from build123d import *

# Parameters (mm, degrees)
F0_W     = 48.26
F0_H     = 73.66
F1_DEPTH = 48.26
F3_DEPTH = 30.48
F5_DEPTH = 30.48
F7_DEPTH = 25.4
F8_W     = 3.175
F8_H     = 3.175
F9_DEPTH = 19.05


with BuildPart() as f1:
    # F0 (on Top) → F1 (new body)
    with BuildSketch(Plane.XY):
        with Locations((24.13, 36.83)):
            Rectangle(F0_W, F0_H)
    extrude(amount=F1_DEPTH)

    # F2 (on face) → F3 (join)
    with BuildSketch(Plane(origin=(0, 73.66, 0), x_dir=(-1, 0, 0), z_dir=(0, 1, 0))):
        Polygon((-12.1206499105, 44.9308045208), (-24.13, 44.9308045208), (-24.13, 24.13), (-24.13, 9.0534836054), (-48.0858952621, 24.0212186931), (-36.1393500895, 3.3291954792), (-12.1206499105, 3.3291954792), (-0.1112998211, 24.13), align=None)
        Polygon((-24.13, 24.13), (-24.13, 44.9308045208), (-36.1393500895, 44.9308045208), (-48.1487001789, 24.13), align=None)
        Polygon((-24.13, 9.0534836054), (-24.13, 24.13), (-48.1487001789, 24.13), (-48.0858952621, 24.0212186931), align=None)
        Polygon((-48.0858952621, 24.0212186931), (-48.1487001789, 24.13), (-48.26, 24.13), align=None)
    extrude(amount=F3_DEPTH)

    # F4 (on face) → F5 (join)
    with BuildSketch(Plane(origin=(0, 104.14, 0), x_dir=(-1, 0, 0), z_dir=(0, 1, 0))):
        Polygon((-15.8659655868, 38.4132767837), (-24.13, 38.4209016232), (-24.13, 24.0781502233), (-7.6297935663, 24.1173632016), align=None)
        Polygon((-24.13, 24.0781502233), (-24.13, 38.4209016232), (-32.3676633374, 38.4285021314), (-40.6316977506, 24.1452253477), (-40.5705446588, 24.0390790321), align=None)
        Polygon((-7.6297935663, 24.1173632016), (-24.13, 24.0781502233), (-24.13, 9.8390983768), (-15.8923366626, 9.8314978686), (-7.6283022494, 24.1147746523), align=None)
        Polygon((-24.13, 9.8390983768), (-24.13, 24.0781502233), (-40.5705446588, 24.0390790321), (-32.3940344132, 9.8467232163), align=None)
    extrude(amount=F5_DEPTH)

    # F6 (on face) → F7 (join)
    with BuildSketch(Plane(origin=(0, 134.62, 0), x_dir=(-1, 0, 0), z_dir=(0, 1, 0))):
        Polygon((-18.9955281103, 33.1531956374), (-24.1168144621, 33.1211234563), (-24.1168144621, 24.1299878343), (-13.7908709872, 24.1204605673), (-13.7484474098, 24.1950147272), align=None)
        Polygon((-24.1168144621, 24.1299878343), (-24.1168144621, 33.1211234563), (-29.3770807004, 33.0881809102), (-34.4691290128, 24.1395394327), align=None)
        Polygon((-13.7908709872, 24.1204605673), (-24.1168144621, 24.1299878343), (-24.1168144621, 15.1390416932), (-18.8829192996, 15.1718190898), align=None)
        Polygon((-24.1168144621, 15.1390416932), (-24.1168144621, 24.1299878343), (-34.4691290128, 24.1395394327), (-34.5115525902, 24.0649852728), (-29.2644718897, 15.1068043626), align=None)
    extrude(amount=F7_DEPTH)

    # F8 (on face) → F9 (join)
    with BuildSketch(Plane.XZ):
        Polygon((40.005, 40.005), (36.83, 40.005), (36.83, 36.83), (36.83, 33.655), (40.005, 33.655), align=None)
        Polygon((36.83, 36.83), (36.83, 40.005), (33.655, 40.005), (33.655, 33.655), (36.83, 33.655), align=None)
        Polygon((8.255, 33.655), (11.43, 33.655), (14.605, 33.655), (14.605, 40.005), (8.255, 40.005), align=None)
        Polygon((14.605, 8.255), (14.605, 11.43), (11.43, 11.43), (11.43, 14.605), (8.255, 14.605), (8.255, 8.255), align=None)
        with Locations((13.0175, 13.0175)):
            Rectangle(F8_W, F8_H)
        Polygon((40.005, 14.605), (36.83, 14.605), (36.83, 11.43), (33.655, 11.43), (33.655, 8.255), (40.005, 8.255), align=None)
        with Locations((35.2425, 13.0175)):
            Rectangle(F8_W, F8_H)
    extrude(amount=F9_DEPTH)


solid = f1.part
Can you work these out from the model? Positions are in its coordinate system, mm. A direction names the side the tool comes from. Give positions to 0.01 mm unless a question says otherwise; leave off trailing zeros. Loops run counter-clockwise (first coordinate to the right, second up) from the corner with the lowest first, then second, coordinate; pieces in that order, holes last. Notation, with made-up numbers: (70, -3.75) - (94, -3.75) arc R8 ccw to (94, 9.25) - close; hole circle Ø11 at (33.5, 35). An arc over 180 degrees is marked (long way). Return JSON: item names as keys, results as strings.
1. For faces 1 (the face through (6.03, 88.69, 34.38)), 2 (the face through (37, -9, 8.255)), 3 (the face through (14.605, -9, 37)), 4 (the face through (8, 104.14, 29)), which set-ups out of +Z, -Z, +X, -X, +Y, -Y let a thin tool reach every point of the face, with its end or its side?
Output values:
{"face 1": "+Z, -X, +Y", "face 2": "-Z, +X, -X, -Y", "face 3": "+Z, -Z, -Y", "face 4": "+Y"}
2. If I drill on line 1 (Z direction, x = 35, y = -2) (3 decimals); line 2 (Y direction, x = 38, z = 26.5); line 3 (Y direction, x = 29, z = 43), over which ranges is the centre line in solid material (lowest first)?
Output values:
{"line 1": "z = 8.255 to 14.605, 33.655 to 40.005", "line 2": "y = 0 to 134.62", "line 3": "y = 0 to 104.14"}
3. We'd pull the mould along Z, two halves only. Please class faces 5 (the face through (24, 89, 44.931)), 6 (the face through (11, -9, 14.605)), 7 (the face through (37, -9, 33.655)), 8 (the face through (40.005, -9, 11)): +Z half, -Z half, draft (parallel to the pull), parting line (faces both ways), or undercut.
Output values:
{"face 5": "+Z half", "face 6": "undercut", "face 7": "undercut", "face 8": "draft"}
4. I want a section at C-C on x = 5. Please give me the cut outline in (y, z).
Output values:
{"outline": "(0, 0) - (73.66, 0) - (73.66, 15.66) - (104.14, 15.66) - (104.14, 32.6) - (73.66, 32.6) - (73.66, 48.26) - (0, 48.26) - close"}
5. I'm going to push flat-ended pins straight in: pin 1 Ø5 at (x, y) = (10.5, -8.5) entering from -Z (3 decimals); pin 2 Ø8 at (y, z) = (125.5, 20) entering from -X; pin 3 Ø7 at (y, z) = (-6, 37) entering from +X (3 decimals). Where does each tip first touch, or does it pass through?
Output values:
{"pin 1": "stops at z = 8.255", "pin 2": "stops at x = 7.69", "pin 3": "stops at x = 40.005"}
6. I want a section at B-B on z = 6. Please give me the cut outline in (x, y), and give its area (3 significant figures).
Output values:
{"outline": "(0, 0) - (48.26, 0) - (48.26, 73.66) - (37.68, 73.66) - (37.68, 104.14) - (10.58, 104.14) - (10.58, 73.66) - (0, 73.66) - close", "area": "4,380 mm²"}
7. I want a section at D-D on y = 146. Please give me the cut outline in (x, z), and give its area (3 significant figures).
Output values:
{"outline": "(13.75, 24.2) - (18.88, 15.17) - (29.26, 15.11) - (34.51, 24.06) - (29.38, 33.09) - (19, 33.15) - close", "area": "280 mm²"}
8. I want a section at A-A on y = 112. Please give me the cut outline in (x, z).
Output values:
{"outline": "(7.63, 24.11) - (15.89, 9.83) - (32.39, 9.85) - (40.63, 24.15) - (32.37, 38.43) - (15.87, 38.41) - close"}
